Design review of the part built by this model. Coordinates are the model's own, in mm. A direction names the side the tool comes from. Round coordinates to 2 decimals unless told otherwise and drop trailing zeros. Write each loop counter-clockwise with the first axis right and the second up, starting at its lowest first coordinate (ties: lowest second). Pieces come first, ordered by that corner, then holes. Notation, with made-up numbers: (45, 16) -> (100, 16) arc R19 cw to (100, 52) -> close; hole circle Ø7 at (55.25, 69). An arc over 180 degrees is marked (long way). Write item = value, one per line. Start each with the question number.
Item 1: Add section A-A, the plane y = -18. State the section outline as (x, z) points.
Item 2: Add section B-B, the plane x = -40. State the section outline as (y, z) points.
Item 3: Machinability: for faces 1 (the cylindrical face through (-15.42, 5.26, 69.43)), 2 (the cylindrical face through (56.507, 10.053, 29.775)), which of the approach directions +Z, -Z, +X, -X, +Y, -Y give a long, thin tool a straight path to every point of the face, cutting with its end or side? Answer none if there is none.
Item 4: Add section D-D, the plane y = 13.5. State how many separate pieces and enclosed holes the cut face has, then the cut area to 3 significant figures.
Item 5: For pin 1 Ø8 at (x, y) = (-18, 12) entering from -Z; pin 2 Ø8 at (x, z) = (54.99, 31.75) entering from +Y; pin 3 Ø6 at (x, z) = (-43, 9.5) entering from +Y; pin 4 Ø3 at (x, z) = (0, 63.5) entering from +Y, all flat-tipped, find the tip position at first contact; note any pin that passes through.
Item 6: Mouldability with a two-part tool opening along Z and no side actions: class faces 3 (the cylindrical face through (-6.607, -19.765, -29.755)), 4 (the conical face through (-5.592, -13.573, 25.184)), 5 (the flat face through (31, -7.62, -31)), 6 (the cylindrical face through (-52.563, 10.053, 31.21)) as released by +Z, released by -Z, zero draft, split by the parting line, or undercut.
Item 7: Add section C-C, the plane y = -10. State the section outline as (x, z) points.
Item 8: To check wall thickness, follow L1, parallel to X at y = 14, z = -31; L2, parallel to Z at x = 0.5, y = -22.5; L3, parallel to X at y = 8, z = 31.75. State the ranges of each line that lie inside material, in increasing order.
Autodesk Inventor part; units mm, degrees
ref_plane "YZ Plane" through (0, 0, 0) normal (1, 0, 0) x (0, 1, 0)
ref_plane "XZ Plane" through (0, 0, 0) normal (0, 1, 0) x (-1, 0, 0)
ref_plane "XY Plane" through (0, 0, 0) normal (0, 0, 1) x (1, 0, 0)
sketch "Sketch1" plane through (0, 0, 0) normal (0, 0, 1) x (1, 0, 0)
  line L0 (71.12, 17.78) -> (66.548, 17.78)
  line L1 (66.548, 17.78) -> (66.548, -7.62)
  line L2 (66.548, -7.62) -> (71.12, -7.62)
  line L3 (71.12, -7.62) -> (71.12, 17.78)
  line L4 (66.548, -7.62) -> (31.75, -7.62)
  line L5 (31.75, -7.62) -> (31.75, 0)
  line L6 (31.75, 0) -> (66.548, 0)
  line L7 (66.548, 0) -> (66.548, -7.62)
  line L8 (25.4, -13.97) -> (30.48, -13.97)
  line L9 (30.48, -13.97) -> (30.48, -25.4)
  line L10 (30.48, -25.4) -> (25.4, -25.4)
  line L11 (25.4, -25.4) -> (25.4, -13.97)
  line L12 (0, 0) -> (0, -50.8709) construction
  line L13 (25.4, -13.97) -> (31.75, -7.62)
  line L14 (30.48, -13.97) -> (36.83, -7.62)
  dimension "d0" = 142.24
  dimension "d1" = 50.8
  dimension "d2" = 4.572
  dimension "d4" = 6.35
  dimension "d5" = 11.43
  dimension "d6" = 25.4
  dimension "d7" = 45
  dimension "d9" = 5.08
  dimension "d10" = 7.62
revolve "Revolution1" add sketch "Sketch1" angle 360 about axis through (0, 0, 0) along (0, -1, 0)
sketch "Sketch2" plane through (0, 17.78, 0) normal (0, 1, 0) x (1, 0, 0)
  circle A0 centre (0, 0) radius 71.12
  line L0 (0, 0) -> (0, 63.5) construction
  circle A1 centre (0, 63.5) radius 5.08
  dimension "d11" = 63.5
  dimension "d12" = 10.16
extrude "Extrusion1" add sketch "Sketch2" against normal up to surface (17.78 mm away) contours A1
fillet "Fillet1" radius 5.08 2 edges at (4.1584, 8.89, -66.418) (-4.1584, 8.89, -66.418)
pattern_circular "Circular Pattern1" count 6 over 360 about axis through (0, -19.685, 0) along (0, -1, 0) of "Extrusion1", "Fillet1"
thread "Thread1"
sketch "Sketch3" plane through (0, 17.78, 0) normal (0, 1, 0) x (1, 0, 0)
  arc A0 (-4.8815, 62.0939) -> (4.8815, 62.0939) centre (0, 63.5) ccw
  arc A1 (-51.3341, -35.2744) -> (-56.2156, -26.8194) centre (-54.9926, -31.75) ccw
  arc A2 (4.8815, -62.0939) -> (-4.8815, -62.0939) centre (0, -63.5) ccw
  arc A3 (56.2156, -26.8194) -> (51.3341, -35.2744) centre (54.9926, -31.75) ccw
  arc A4 (51.3341, 35.2744) -> (56.2156, 26.8194) centre (54.9926, 31.75) ccw
  arc A5 (-56.2156, 26.8194) -> (-51.3341, 35.2744) centre (-54.9926, 31.75) ccw
  point P0 (0, 63.5)
  point P1 (-51.8006, -35.7019)
  point P2 (-56.819, -27.0097)
  point P3 (5.0184, -62.7116)
  point P4 (-5.0184, -62.7116)
  point P5 (56.819, -27.0097)
  point P6 (51.8006, -35.7019)
  point P7 (51.8006, 35.7019)
  point P8 (56.819, 27.0097)
  point P9 (-56.819, 27.0097)
  point P10 (-51.8006, 35.7019)
hole "Hole1" at (0, 17.78, -63.5) at (-54.9926, 17.78, 31.75) at (0, 17.78, 63.5) at (54.9926, 17.78, 31.75) at (54.9926, 17.78, -31.75) at (-54.9926, 17.78, -31.75) direction (0, -1, 0) diameter 4.9784 depth 15.24 tip angle 118
properties part number "Cap Housing Base"
Result set:
q1.outline = circle Ø60.96 at (0, 0); hole circle Ø50.8 at (0, 0)
q2.outline = (-7.62, -58.81) -> (17.78, -58.81) -> (17.78, -53.18) -> (0, -53.18) -> (0, 53.18) -> (17.78, 53.18) -> (17.78, 58.81) -> (-7.62, 58.81) -> close
q3.face_1 = +Y, -Y
q3.face_2 = +Y
q4.separate_pieces = 1
q4.enclosed_holes = 7
q4.area = 2,350 mm²
q5.pin_1 = -69.73
q5.pin_2 = 17.78
q5.pin_3 = 0
q5.pin_4 = 1.95
q6.face_3 = split by the parting line
q6.face_4 = undercut
q6.face_5 = zero draft
q6.face_6 = undercut
q7.outline = circle Ø68.9 at (0, 0); hole circle Ø58.74 at (0, 0)
q8.L1 = -64.01 to -57.37, -52.62 to -49.97, 49.97 to 52.62, 57.37 to 64.01
q8.L2 = -30.48 to -25.4, 25.4 to 30.48
q8.L3 = -63.64 to -57.48, -52.5 to -49.91, 49.91 to 52.5, 57.48 to 63.64
